Autodesk Inventor part; units mm, degrees
ref_plane "YZ Plane" through (0, 0, 0) normal (1, 0, 0) x (0, 1, 0)
ref_plane "XY Plane" through (0, 0, 0) normal (0, 0, 1) x (1, 0, 0)
sketch "Sketch1" plane through (0, 0, 0) normal (0, 1, 0) x (-1, 0, 0)
  line L0 (25.9, 0) -> (-25.9, 0)
  line L1 (0, -25.9) -> (0, 25.9)
  circle A0 centre (0, 0) radius 18.5 construction
  circle A1 centre (0, 0) radius 13 construction
  dimension "d0" = 37
  dimension "d1" = 26
sketch "Sketch2" plane through (0, 0, 0) normal (0, 1, 0) x (-1, 0, 0)
  line L0 (88.2, 0) -> (-88.2, 0)
  line L1 (0, -36.8) -> (0, 73.8)
  line L2 (-63, 58) -> (-63, -21)
  line L3 (-63, -21) -> (63, -21)
  line L4 (63, -21) -> (63, 58)
  line L5 (-63, 58) -> (63, 58)
  point P0 (0, 0)
  dimension "d3" = 126
  dimension "d29" = 21
  dimension "d30" = 58
extrude "Extrusion1" add sketch "Sketch2" along normal blind 7
sketch "Sketch6" plane through (0, 0, 0) normal (0, 1, 0) x (-1, 0, 0)
  line L0 (63, -21) -> (-63, -21)
  line L1 (63, 58) -> (63, -21)
  line L2 (-63, -21) -> (63, -21)
  line L3 (63, -21) -> (63, 58)
  line L4 (-63, 58) -> (-63, -21)
  line L5 (88.2, 0) -> (-88.2, 0)
  line L6 (0, -36.3) -> (0, 70.8)
  line L7 (63, 58) -> (-63, 58)
  line L8 (-53, 58) -> (-53, 0)
  line L9 (53, 0) -> (53, 58)
  line L10 (53, 58) -> (63, 58)
  line L11 (-63, 58) -> (-63, -21)
  line L12 (-63, 58) -> (-53, 58)
  arc A0 (37, -16) -> (53, 0) centre (37, 0) ccw
  arc A1 (-53, 0) -> (-37, -16) centre (-37, 0) ccw
  line L13 (37, -16) -> (-39.8141, -16)
  point P0 (0, 0)
  point P1 (-16, 0)
  dimension "d101" = 53
  dimension "d102" = 53
  dimension "d103" = 32
  dimension "d104" = 32
extrude "Extrusion5" add sketch "Sketch6" against normal blind 5.5 contours L0 L6 L13 A0 L5 L1 | L0 L4 L5 A1 L13 L6 | L5 L9 L7 L1 | L4 L7 L8 L5
sketch "Sketch4" plane through (0, 0, 0) normal (0, 0, 1) x (1, 0, 0)
  line L0 (-55.5, 0) -> (55.5, 0)
  line L1 (55.5, 0) -> (55.5, -2.5)
  line L2 (55.5, -2.5) -> (-55.5, -2.5)
  line L3 (-55.5, -2.5) -> (-55.5, 0)
  line L4 (-77.7, 0) -> (77.7, 0)
  line L5 (0, -3) -> (0, 0.5)
  point P0 (0, 0)
  dimension "d10" = 111
  dimension "d11" = 2.5
extrude "Extrusion6" cut sketch "Sketch4" against normal blind 21
sketch "Sketch5" plane through (0, 0, 0) normal (0, 1, 0) x (-1, 0, 0)
  circle A0 centre (0, 0) radius 18.5 construction
  circle A1 centre (0, 0) radius 18.5 construction
  line L0 (77.7, 0) -> (-77.7, 0)
  line L1 (0, -28.9) -> (0, 26.4)
  line L2 (-55.5, -21) -> (55.5, -21)
  line L3 (55.5, -21) -> (55.5, -18.5)
  line L4 (55.5, -18.5) -> (-55.5, -18.5)
  line L5 (-55.5, -18.5) -> (-55.5, -21)
  dimension "d25" = 111
  dimension "d26" = 21
extrude "Extrusion7" add sketch "Sketch5" against normal blind 2.5
sketch "Sketch7" plane through (0, 0, 0) normal (0, 0, 1) x (1, 0, 0)
  line L0 (-55.5, 0) -> (55.5, 0)
  line L1 (55.5, 0) -> (55.5, -2.5)
  line L2 (55.5, -2.5) -> (-55.5, -2.5)
  line L3 (-55.5, -2.5) -> (-55.5, 0)
  line L4 (53, 0) -> (-53, 0)
  line L5 (-77.7, 0) -> (77.7, 0)
  line L6 (0, -3) -> (0, 0.5)
  point P0 (-16, 0)
  point P1 (16, 0)
  dimension "d53" = 2.5
  dimension "d54" = 55.5
extrude "Extrusion8" cut sketch "Sketch7" along normal blind 58
sketch "Sketch8" plane through (0, 0, 0) normal (0, 1, 0) x (-1, 0, 0)
  circle A0 centre (0, 0) radius 13
  dimension "d34" = 26
extrude "Extrusion9" cut sketch "Sketch8" along normal through all
pattern_linear "Rectangular Pattern1" count 2 spacing 37 along (0, 0, 1) count 3 spacing 37 along (1, 0, 0) of "Extrusion9" second direction both ways yes
sketch "Sketch9" plane through (0, 7, 0) normal (0, 1, 0) x (1, 0, 0)
  circle A0 centre (0, 0) radius 13
  circle A1 centre (0, 0) radius 15
  dimension "d40" = 26
  dimension "d41" = 30
extrude "Extrusion10" [suppressed]
sketch "Sketch10" plane through (0, 5, 0) normal (0, 1, 0) x (1, 0, 0)
  arc A0 (16, 0) -> (-16, 0) centre (0, 0) ccw
  line L0 (1.5, -18) -> (-1.5, -18)
  line L1 (-29.4, 0) -> (29.4, 0)
  line L2 (0, 36.3) -> (0, -70.8)
  line L3 (1.5, -12) -> (-1.5, -12)
  line L4 (1.5, -12) -> (1.5, -18)
  line L5 (-1.5, -18) -> (-1.5, -12)
  dimension "d48" = 3
  dimension "d49" = 12
  dimension "d50" = 6
extrude "Extrusion11" [suppressed]
ref_plane "Work Plane1" through (0, 5, 0) normal (0, 1, 0) x (-1, 0, 0)
sketch "Sketch12" plane through (0, 5, 0) normal (0, 1, 0) x (-1, 0, 0)
  line L0 (63, 58) -> (63, -21)
  line L1 (63, -21) -> (-63, -21)
  line L2 (-63, -21) -> (-63, -51)
  line L3 (-63, -51) -> (63, -51)
  line L4 (63, -51) -> (63, -21)
  point P0 (0, 0)
  dimension "d61" = 126
  dimension "d62" = 30
extrude "Extrusion12" add sketch "Sketch12" against normal blind 34.5
sketch "Sketch13" plane through (0, 0, 0) normal (1, 0, 0) x (0, 1, 0)
  line L0 (-31.4, 0) -> (13.4, 0)
  line L1 (0, -62.5) -> (0, 32)
  line L2 (7, -19) -> (7, -49)
  line L3 (7, -49) -> (-25, -43.3575)
  line L4 (-25, -43.3575) -> (-25, -30.647)
  line L5 (7, -19) -> (-25, -30.647)
  point P0 (0, 0)
  dimension "d85" = 25
  dimension "d86" = 7
  dimension "d87" = 49
  dimension "d88" = 30
  dimension "d89" = 100
  dimension "d90" = 110
extrude "Extrusion14" cut sketch "Sketch13" along normal mid plane 122
sketch "Sketch14" plane through (0, 5, 0) normal (0, 1, 0) x (-1, 0, 0)
  line L0 (0, -72.3) -> (0, 76.8)
  line L1 (61, 56) -> (-61, 56)
  line L2 (-61, 56) -> (-61, -49)
  line L3 (-61, -49) -> (61, -49)
  line L4 (61, -49) -> (61, 56)
  line L5 (63, 58) -> (-63, 58)
  line L6 (-63, 58) -> (-63, -51)
  line L7 (-63, -51) -> (63, -51)
  line L8 (63, -51) -> (63, 58)
  line L9 (88.2, 0) -> (-88.2, 0)
  dimension "d91" = 51
  dimension "d92" = 58
  dimension "d93" = 126
  dimension "d94" = 122
  dimension "d95" = 56
  dimension "d96" = 49
extrude "Extrusion15" add sketch "Sketch14" along normal blind 10 contours L7 L6 L9 L2 L3 L0 | L0 L3 L4 L9 L8 L7 | L6 L5 L0 L1 L2 L9 | L9 L4 L1 L0 L5 L8
fillet "Fillet3" radius 2 4 edges at (63, 4.75, 58) (63, -7.25, -51) (-63, -7.25, -51) (-63, 4.75, 58)
fillet "Fillet5" radius 2 2 edges at (63, -17.5, -21) (-63, -17.5, -21)
fillet "Fillet6" radius 2 2 edges at (0, 7, 56) (0, 7, -19)
fillet "Fillet7" radius 4 2 edges at (0, -25, -30.647) (0, -25, -43.3575)
fillet "Fillet8" radius 2 2 edges at (-53, -4, 58) (53, -4, 58)
equation "\"d102\" = d101"
properties part number "NespressoSpeedfiller-6X"
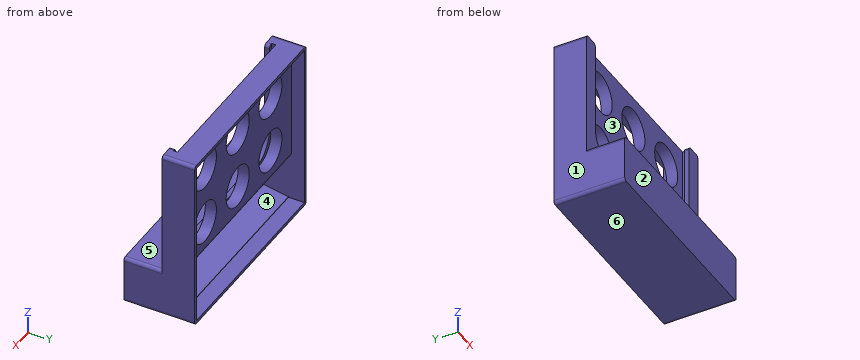
Source: CAD feature listing. Evaluate the final solid. Frame: model axes, mm. Face numbers are marked on the shaded views. A direction names the side the tool comes from. Round coordinates to 2 decimals unless told otherwise and drop trailing zeros. Order: outer loops, then holes, each group sorted by start corner. A loop starts at its lowest first (then second) coordinate and runs counter-clockwise, first axis right, second up. Notation, with made-up numbers: (-35.75, 53.25) -> (23.25, 53.25) arc R27 cw to (23.25, 77.25) -> close; hole circle Ø10 at (76.25, 32). An arc over 180 degrees is marked (long way). Answer as CSV lines item,"result".
Item 1: Section A-A, the plane x = 0. Count the separate pieces of the cut face and the enclosed holes in it, plus the area to 3 significant figures.
A:
separate pieces,"3"
enclosed holes,"0"
area,"658 mm²"
Item 2: Pull-direction query (X, two-part tool) for the marked faces 1, 2 and 3; classes: pulls with the +X half, pulls with the -X half, needs draft (parallel to the pull), parting line crosses it, or undercut.
A:
face 1,"pulls with the -X half"
face 2,"needs draft"
face 3,"undercut"
Item 3: Line query: L1, parallel to X at y = 2, z = 37; L2, parallel to X at y = 7, z = -42; L3, parallel to Z at x = 0, y = 3. Output: solid intervals per line, ascending.
A:
L1,"-63 to -50, -24 to -13, 13 to 24, 50 to 63"
L2,"-63 to -61, 61 to 63"
L3,"-51 to -48.29, -20.46 to -13, 13 to 24, 50 to 58"
Item 4: Pin query (flat end, axial travel): pin 1 Ø1 at (x, z) = (19.5, 13) entering from +Y; pin 2 Ø2.5 at (x, y) = (16.5, -4) entering from +Z; pin 3 Ø0.8 at (x, y) = (17.5, -1.5) entering from +Z. Return the tip coordinate at first contact, or that it passes through.
A:
pin 1,"y = 7"
pin 2,"z = -16"
pin 3,"z = -18.5"
Item 5: Section D-D, the plane z = -42.5. Return loops of the section in (x, y), plus the area to 3 significant figures.
A:
outline,"(-63, -29.5) -> (63, -29.5) -> (63, 15) -> (61, 15) -> (61, -24.12) -> (-61, -24.12) -> (-61, 15) -> (-63, 15) -> close"
area,"834 mm²"
Item 6: Section B-B, the plane z = 37. Return loops of the section in (x, y).
A:
outline,"(-63, -5.5) -> (-53, -5.5) -> (-53, -2.5) -> (-55.5, -2.5) -> (-55.5, 0) -> (-50, 0) -> (-50, 7) -> (-61, 7) -> (-61, 15) -> (-63, 15) -> close; (-24, 0) -> (-13, 0) -> (-13, 7) -> (-24, 7) -> close; (13, 0) -> (24, 0) -> (24, 7) -> (13, 7) -> close; (50, 0) -> (55.5, 0) -> (55.5, -2.5) -> (53, -2.5) -> (53, -5.5) -> (63, -5.5) -> (63, 15) -> (61, 15) -> (61, 7) -> (50, 7) -> close"
Item 7: Reachability of the marked faces 4, 5 and 6 from +Z, -Z, +X, -X, +Y, -Y: full face, straight path, thin tool, end or side. Return the list, or none.
A:
face 4,"+Y"
face 5,"+Z, +X, -X, -Y"
face 6,"-Z, +X, -X, +Y, -Y"
